Could you check a few things on this model? Use its own coordinates, in mm. A direction names the side the tool comes from. Round coordinates to 2 decimals unless told otherwise and drop trailing zeros. Loops run counter-clockwise (first coordinate to the right, second up) from the corner with the lowest first, then second, coordinate; pieces in that order, holes last.
from build123d import *

# Parameters (mm, degrees)
BOSS_EXTRUDE1_DEPTH = 15


with BuildPart() as part:
    # Sketch1 → Boss-Extrude1 (new, symmetric)
    with BuildSketch(Plane.XY):
        with BuildLine():
            Line((-299.814682012, 198.540409756), (-139.331537098, 105.88542284))
            ThreePointArc((-139.331537098, 105.88542284), (-87.5, 151.554445662), (-22.033697521, 173.607362095))
            Line((-22.033697521, 173.607362095), (-22.033697521, 358.917335928))
            ThreePointArc((-22.033697521, 358.917335928), (0, 380.951033449), (22.033697521, 358.917335928))
            Line((22.033697521, 358.917335928), (22.033697521, 173.607362095))
            ThreePointArc((22.033697521, 173.607362095), (87.5, 151.554445662), (139.331537098, 105.88542284))
            Line((139.331537098, 105.88542284), (299.814682012, 198.540409756))
            ThreePointArc((299.814682012, 198.540409756), (329.913272565, 190.475516725), (321.848379533, 160.376926172))
            Line((321.848379533, 160.376926172), (161.365234619, 67.721939255))
            ThreePointArc((161.365234619, 67.721939255), (175, 0), (161.365234619, -67.721939255))
            Line((161.365234619, -67.721939255), (321.848379533, -160.376926172))
            ThreePointArc((321.848379533, -160.376926172), (329.913272565, -190.475516725), (299.814682012, -198.540409756))
            Line((299.814682012, -198.540409756), (139.331537098, -105.88542284))
            ThreePointArc((139.331537098, -105.88542284), (87.5, -151.554445662), (22.033697521, -173.607362095))
            Line((22.033697521, -173.607362095), (22.033697521, -358.917335928))
            ThreePointArc((22.033697521, -358.917335928), (0, -380.951033449), (-22.033697521, -358.917335928))
            Line((-22.033697521, -358.917335928), (-22.033697521, -173.607362095))
            ThreePointArc((-22.033697521, -173.607362095), (-87.5, -151.554445662), (-139.331537098, -105.88542284))
            Line((-139.331537098, -105.88542284), (-299.814682012, -198.540409756))
            ThreePointArc((-299.814682012, -198.540409756), (-329.913272565, -190.475516725), (-321.848379533, -160.376926172))
            Line((-321.848379533, -160.376926172), (-161.365234619, -67.721939255))
            ThreePointArc((-161.365234619, -67.721939255), (-175, 0), (-161.365234619, 67.721939255))
            Line((-161.365234619, 67.721939255), (-321.848379533, 160.376926172))
            ThreePointArc((-321.848379533, 160.376926172), (-329.913272565, 190.475516725), (-299.814682012, 198.540409756))
        make_face()
    extrude(amount=BOSS_EXTRUDE1_DEPTH, both=True)


solid = part.part
Item 1: If we section it at D-D, the plane y = -299: Please give me the cut outline in (x, z).
Results list:
outline: (-22.03, -15) - (22.03, -15) - (22.03, 15) - (-22.03, 15) - close
Item 2: If we section it at C-C, the plane z = 9.25: Please give me the cut outline in (x, y).
Results list:
outline: (-321.85, -160.38) arc R22.03 ccw to (-299.81, -198.54) - (-139.33, -105.89) arc R175 ccw to (-22.03, -173.61) - (-22.03, -358.92) arc R22.03 ccw to (22.03, -358.92) - (22.03, -173.61) arc R175 ccw to (139.33, -105.89) - (299.81, -198.54) arc R22.03 ccw to (321.85, -160.38) - (161.37, -67.72) arc R175 ccw to (161.37, 67.72) - (321.85, 160.38) arc R22.03 ccw to (299.81, 198.54) - (139.33, 105.89) arc R175 ccw to (22.03, 173.61) - (22.03, 358.92) arc R22.03 ccw to (-22.03, 358.92) - (-22.03, 173.61) arc R175 ccw to (-139.33, 105.89) - (-299.81, 198.54) arc R22.03 ccw to (-321.85, 160.38) - (-161.37, 67.72) arc R175 ccw to (-161.37, -67.72) - close
Item 3: If we section it at B-B, the plane y = 119: Please give me the cut outline in (x, z).
Results list:
outline: (-250.18, -15) - (-162.05, -15) - (-162.05, 15) - (-250.18, 15) - close; (-128.31, -15) - (128.31, -15) - (128.31, 15) - (-128.31, 15) - close; (162.05, -15) - (250.18, -15) - (250.18, 15) - (162.05, 15) - close
Item 4: We'd pull the mould along X, two halves only. Please class faces 1 (the cylindrical face through (-174.997, -0.974, 0.21)), 2 (the cylindrical face through (0.485, -380.946, 0.21)), 3 (the cylindrical face through (-88.342, 151.065, 0.21)): released by +X, released by -X, zero draft, split by the parting line, or undercut.
Results list:
face 1: released by -X
face 2: split by the parting line
face 3: undercut
Item 5: If I drill on line 1 along X through (y, z) = (-339, -9); line 2 along X through (y, z) = (-148, 13); line 3 along Y through (x, z) = (183.5, 10), over which ranges is the centre line in solid material (lowest first)?
Results list:
line 1: x = -22.03 to 22.03
line 2: x = -300.41 to -212.28, -93.39 to 93.39, 212.28 to 300.41
line 3: y = -131.39 to -80.5, 80.5 to 131.39
Item 6: Will these pins go through, and if not, where does the flat tip stop? pin 1 (15 mm diameter, centred on y = 280, z = 3.5, fed in from +X); pin 2 (3 mm diameter, centred on y = -85, z = 3.5, fed in from +X); pin 3 (8 mm diameter, centred on x = 64.5, z = 9, fed in from +Y).
Results list:
pin 1: stops at x = 22.03
pin 2: stops at x = 193.89
pin 3: stops at y = 164.21
Item 7: For faces 4 (the cylindrical face through (-86.656, -152.039, 0.21)), 5 (the flat face through (-242.73, -114.7, 0.21)), 6 (the flat face through (240.48, -113.4, 0.21)), 7 (the flat face through (218.45, 151.564, 0.21)), which set-ups out of +Z, -Z, +X, -X, +Y, -Y let a thin tool reach every point of the face, with its end or its side?
Results list:
face 4: +Z, -Z, -Y
face 5: +Z, -Z, -X
face 6: +Z, -Z, +X
face 7: +Z, -Z, +Y
Item 8: If we section it at A-A, the plane x = -254: Please give me the cut outline in (y, z), then the cut area to 3 significant figures.
Results list:
outline: (-172.09, -15) - (-121.2, -15) - (-121.2, 15) - (-172.09, 15) - close; (121.2, -15) - (172.09, -15) - (172.09, 15) - (121.2, 15) - close
area: 3,050 mm2
